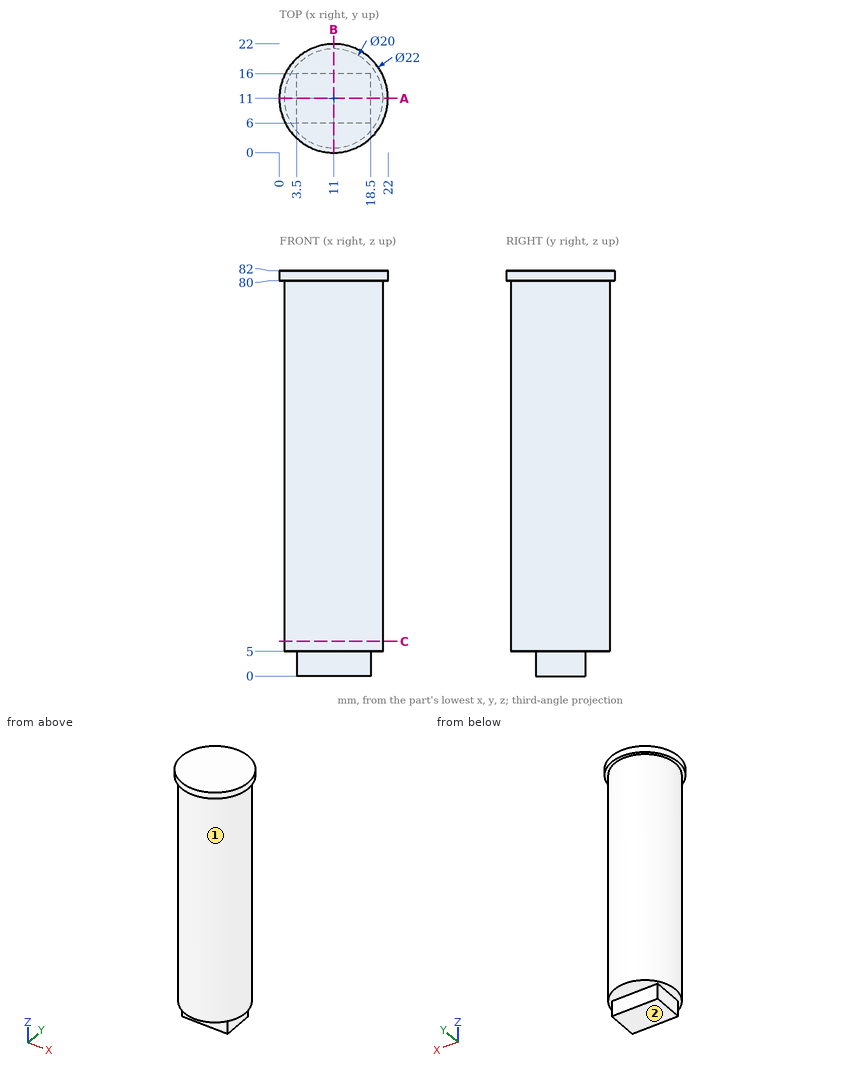
For this review, use the dimensioned drawing (mm, ordinates from the lowest corner) and the shaded views. A direction names the side the tool comes from. Coordinates: 2 decimals unless noted, no trailing zeros. Write each loop counter-clockwise with the first axis right and the second up, starting at its lowest first coordinate (ties: lowest second). Pieces come first, ordered by that corner, then holes. Notation, with made-up numbers: (-25.75, -28.75) -> (-7.75, -28.75) arc R9 ccw to (-7.75, -17.75) -> close; hole circle Ø5 at (8.25, -36). An arc over 180 degrees is marked (long way). Put each result on its own line as item: value.
Q1. Tool access review of the marked faces 1 and 2: name each direction out of +Z, -Z, +X, -X, +Y, -Y from which nothing blocks a thin tool from reaching the whole face with its end or side.
From the geometry:
face 1: -Z
face 2: -Z, +X, -X, +Y, -Y
Q2. Take a section at A-A, the plane y = 11. State the section outline as (x, z) points.
From the geometry:
outline: (0, 80) -> (1, 80) -> (1, 5) -> (3.5, 5) -> (3.5, 0) -> (18.5, 0) -> (18.5, 5) -> (21, 5) -> (21, 80) -> (22, 80) -> (22, 82) -> (0, 82) -> close
Q3. Take a section at C-C, the plane z = 7. State the section outline as (x, y) points.
From the geometry:
outline: circle Ø20 at (11, 11)
Q4. Take a section at B-B, the plane x = 11. State the section outline as (y, z) points, then the cut area to 3 significant figures.
From the geometry:
outline: (0, 80) -> (1, 80) -> (1, 5) -> (6, 5) -> (6, 0) -> (16, 0) -> (16, 5) -> (21, 5) -> (21, 80) -> (22, 80) -> (22, 82) -> (0, 82) -> close
area: 1,590 mm2
Q5. Clearance check with flat-ended pins moving along their axes: pin 1 Ø1.5 at (y, z) = (10, 1.5) entering from -X; pin 2 Ø8 at (y, z) = (11.5, 43) entering from -X; pin 3 Ø6 at (x, z) = (13.5, 67.5) entering from +Y. State where each tip first meets the part, or that it passes through.
From the geometry:
pin 1: stops at x = 3.5
pin 2: stops at x = 1
pin 3: stops at y = 21
Q6. Wall thickness on L1, parallel to Z at x = 16.25, y = 1.75; L2, parallel to Z at x = 2.75, y = 11.5; L3, parallel to Y at x = 11.25, z = 75: over which ranges is each line inside the solid? List them lowest first.
From the geometry:
L1: z = 80 to 82
L2: z = 5 to 82
L3: y = 1 to 21
